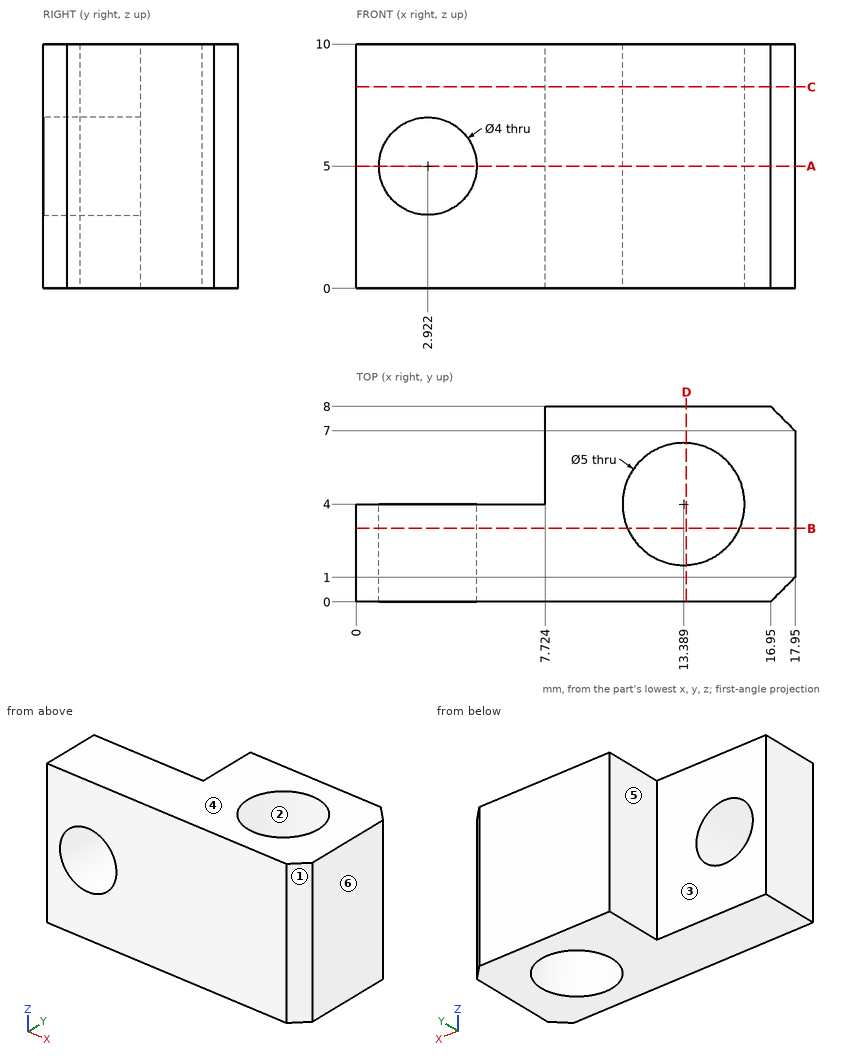
Can you work these out from the drawing? Everything is in mm from the part's minimum corner. A direction names the side the tool comes from. Round coordinates to 2 decimals unless told otherwise and drop trailing zeros. Loops run counter-clockwise (first coordinate to the right, second up) from the corner with the lowest first, then second, coordinate; pieces in that order, holes last. Notation, with made-up numbers: (83, -29) -> (105, -29) arc R16 cw to (105, -9) -> close; hole circle Ø10 at (-28.75, 61). An arc over 180 degrees is marked (long way). Put each result on its own line as item: value.
Q1. Which directions (+Z, -Z, +X, -X, +Y, -Y) give clear straight access to the entire face, cutting with the end or side of a thin tool? Please do the marked faces 5 and 6.
Checks:
face 5: +Z, -Z, -X, +Y
face 6: +Z, -Z, +X, +Y, -Y
Q2. For pin 1 Ø3 at (y, z) = (6, 7.5) entering from -X; pin 2 Ø2 at (x, y) = (13.5, 4) entering from -Z, each with a flat end and sliding along its axis, tell me the tip position at first contact or that it passes through.
Checks:
pin 1: x = 7.72
pin 2: through
Q3. Please list where these lines run through material, in increasing order: line 1 (Y direction, x = 13.25, z = 6.25); line 2 (X direction, y = 1.1, z = 5); line 3 (X direction, y = 6.75, z = 9.75). Write a range as from..to.
Checks:
line 1: 0..1.5, 6.5..8
line 2: 0..0.92, 4.92..17.95
line 3: 7.72..17.95
Q4. I want a section at D-D on x = 13.5. Write out the boundary of the cut face in (y, z).
Checks:
outline: (0, 0) -> (1.5, 0) -> (1.5, 10) -> (0, 10) -> close; (6.5, 0) -> (8, 0) -> (8, 10) -> (6.5, 10) -> close
Q5. I want a section at A-A on z = 5. Write out the boundary of the cut face in (x, y).
Checks:
outline: (0, 0) -> (0.92, 0) -> (0.92, 4) -> (0, 4) -> close; (4.92, 0) -> (16.95, 0) -> (17.95, 1) -> (17.95, 7) -> (16.95, 8) -> (7.72, 8) -> (7.72, 4) -> (4.92, 4) -> close; hole circle Ø5 at (13.39, 4)
Q6. I want a section at C-C on z = 8.25. Write out the boundary of the cut face in (x, y).
Checks:
outline: (0, 0) -> (16.95, 0) -> (17.95, 1) -> (17.95, 7) -> (16.95, 8) -> (7.72, 8) -> (7.72, 4) -> (0, 4) -> close; hole circle Ø5 at (13.39, 4)
Q7. I want a section at B-B on y = 3. Write out the boundary of the cut face in (x, z).
Checks:
outline: (0, 0) -> (11.1, 0) -> (11.1, 10) -> (0, 10) -> close; (15.68, 0) -> (17.95, 0) -> (17.95, 10) -> (15.68, 10) -> close; hole circle Ø4 at (2.92, 5)
Q8. Thinking about a two-plate mould opening in Y: for the marked faces 1, 2, 3 and 4, which applies, pulls with the +Y half, pulls with the -Y half, needs draft (parallel to the pull), parting line crosses it, or undercut?
Checks:
face 1: pulls with the -Y half
face 2: undercut
face 3: pulls with the +Y half
face 4: needs draft
